Build history of the part. All positions in model axes, mm. Round coordinates to 2 decimals unless told otherwise and drop trailing zeros. Write each loop counter-clockwise with the first axis right and the second up, starting at its lowest first coordinate (ties: lowest second). Pieces come first, ordered by that corner, then holes.
Item 1: Wall check: probe 1 along X at (y, z) = (4.6, -8.89); probe 2 along X at (y, z) = (2.7, -7.25); probe 3 along X at (y, z) = (1.75, -17.25). Give the ranges that are in metal, low to high.
Item 2: Band-saw the part on B-B, the plane x = 12.7. Write the cut outline in (y, z) (3 decimals), then the cut area to 3 significant figures.
Item 3: Band-saw the part on A-A, the plane z = -8.89. Write the cut outline in (x, y) (3 decimals).
Item 4: Mould opens along Z. For faces 1 (the cylindrical face through (75.818, 2.88, -0.362)), 2 (the cylindrical face through (0.382, 0.362, -9.319)), 3 (the flat face through (13, 2.54, -9)), 4 (the flat face through (38, 3, -18.415)) say: +Z half, -Z half, draft (parallel to the pull), parting line (faces both ways), or undercut.
```python
from build123d import *

# Parameters (mm, degrees)
SKETCH1_W           = 18.415
SKETCH1_H           = 5.715
BOSS_EXTRUDE1_DEPTH = 76.2
SKETCH2_R           = 2.54
CUT_EXTRUDE1_DEPTH  = 3.175
FILLET1_R           = 1.27


with BuildPart() as part:
    # Sketch1 → Boss-Extrude1 (new body)
    with BuildSketch(Plane(origin=(0, 0, 0), x_dir=(0, 0, -1), z_dir=(1, 0, 0))):
        with Locations((9.2075, 2.8575)):
            Rectangle(SKETCH1_W, SKETCH1_H)
    extrude(amount=BOSS_EXTRUDE1_DEPTH)

    # Sketch2 → Cut-Extrude1 (cut)
    with BuildSketch(Plane(origin=(0, 5.715, 0), x_dir=(1, 0, 0), z_dir=(0, 1, 0))):
        with Locations(Location((12.7, 8.89, 0), (0, 0, 270))):
            Circle(SKETCH2_R)
    extrude(amount=-CUT_EXTRUDE1_DEPTH, mode=Mode.SUBTRACT)

    # Fillet1
    fillet1_edges = [part.edges().sort_by_distance(p)[0] for p in [
        (76.2, 2.8575, -18.415),
        (76.2, 5.715, -9.2075),
        (76.2, 2.8575, 0),
        (0, 5.715, -9.2075),
        (0, 2.8575, -18.415),
        (0, 0, -9.2075),
        (0, 2.8575, 0),
        (38.1, 5.715, 0),
        (38.1, 5.715, -18.415),
        (38.1, 0, -18.415),
        (38.1, 0, 0),
        (76.2, 0, -9.2075),
    ]]
    fillet(fillet1_edges, radius=FILLET1_R)


solid = part.part
```
Results:
1. probe 1: x = 0.01 to 10.16, 15.24 to 76.19
1. probe 2: x = 0 to 10.76, 14.64 to 76.2
1. probe 3: x = 0 to 76.2
2. outline: (0, -17.145) arc R1.27 ccw to (1.27, -18.415) - (4.445, -18.415) arc R1.27 ccw to (5.715, -17.145) - (5.715, -11.43) - (2.54, -11.43) - (2.54, -6.35) - (5.715, -6.35) - (5.715, -1.27) arc R1.27 ccw to (4.445, 0) - (1.27, 0) arc R1.27 ccw to (0, -1.27) - close
2. area: 87.7 mm2
3. outline: (0, 1.27) arc R1.27 ccw to (1.27, 0) - (74.93, 0) arc R1.27 ccw to (76.2, 1.27) - (76.2, 4.445) arc R1.27 ccw to (74.93, 5.715) - (15.24, 5.715) - (15.24, 2.54) - (10.16, 2.54) - (10.16, 5.715) - (1.27, 5.715) arc R1.27 ccw to (0, 4.445) - close
4. face 1: +Z half
4. face 2: draft
4. face 3: undercut
4. face 4: -Z half
